Check sheet for the modelled part. Datum: model origin and axes. Units: mm. Face numbers are marked on the shaded views. Coordinates: 2 decimals unless noted, no trailing zeros. Loops run counter-clockwise (first coordinate to the right, second up) from the corner with the lowest first, then second, coordinate; pieces in that order, holes last. Notation, with made-up numbers: (-28.5, 41) - (5.5, 41) arc R18 ccw to (5.5, 58) - close; hole circle Ø8 at (19.25, 66.5). An arc over 180 degrees is marked (long way). Write each question's results on one line, items separated by ' | '. Start each with the question number.
1. Draft check along X on the marked faces 1, 2, 3 and 4. Enter one of: released by +X, released by -X, zero draft, split by the parting line, or undercut.
2. Cross-section at D-D (x = -6). Record the cut outline in (y, z), and give its area (3 significant figures).
3. Gauge pin test, flat ends, axial feed: P1, Ø1.5, axis at x = 10, z = -16.5, coming from the -Y side; P2, Ø3, axis at x = 3, z = 10.5, coming from the -Y side; P3, Ø4, axis at x = -10, z = 13, coming from the -Y side. Record the tip position at first contact, or that the pin passes through.
4. Thickness scan on line 1 (Z direction, x = 14, y = 6); line 2 (Y direction, x = 0, z = 0.5); line 3 (Y direction, x = 0, z = 17). Record the ranges inside material, lowest first. Write a range as [from, to].
5. Cross-section at C-C (z = 15). Record the cut outline in (x, y), and give its area (3 significant figures).
6. Cross-section at A-A (x = 0). Record the cut outline in (y, z).
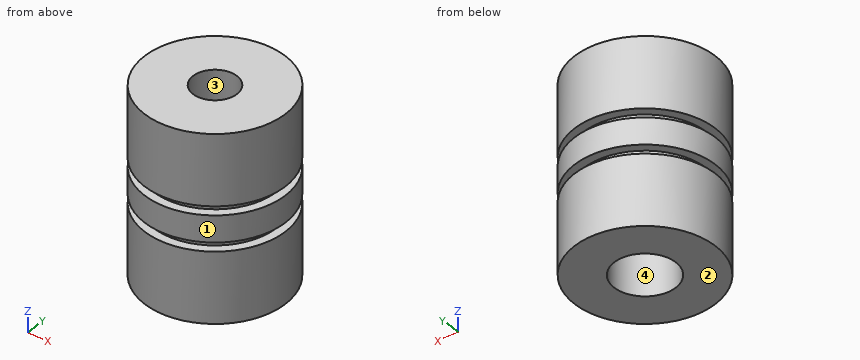
```python
from build123d import *

# Parameters (mm, degrees)
SKETCH_1_R          = 16
SKETCH_1_R_2        = 5
EXTRUDE_1_DEPTH     = 21
SKETCH_2_R          = 7
CUT_EXTRUDE_1_DEPTH = 30
CUT_EXTRUDE_START   = 5
SKETCH_3_R          = 16
SKETCH_3_R_2        = 14
CUT_EXTRUDE_3_DEPTH = 2
CUT_EXTRUDE_START_2 = -3
SKETCH_3_2_R        = 16
SKETCH_3_2_R_2      = 14
CUT_EXTRUDE_4_DEPTH = 2


with BuildPart() as part:
    # Sketch 1 → Extrude 1 (new, symmetric)
    with BuildSketch(Plane.XY):
        with Locations(Location((0, 0, 0), (0, 0, 180))):
            Circle(SKETCH_1_R)
        with Locations(Location((0, 0, 0), (0, 0, 180))):
            Circle(SKETCH_1_R_2, mode=Mode.SUBTRACT)
    extrude(amount=EXTRUDE_1_DEPTH, both=True)

    # Sketch 2 → Cut-Extrude 1 (cut)
    with BuildSketch(Plane(origin=(0, 0, -21), x_dir=(-1, 0, 0), z_dir=(0, 0, -1))):
        Circle(SKETCH_2_R)
    extrude(amount=-CUT_EXTRUDE_1_DEPTH, mode=Mode.SUBTRACT)

    # Sketch 3 → Cut-Extrude 3 (cut)
    with BuildSketch(Plane.XY.offset(CUT_EXTRUDE_START)):
        with Locations(Location((0, 0, 0), (0, 0, 180))):
            Circle(SKETCH_3_R)
        Circle(SKETCH_3_R_2, mode=Mode.SUBTRACT)
    extrude(amount=-CUT_EXTRUDE_3_DEPTH, mode=Mode.SUBTRACT)

    # Sketch 3_2 → Cut-Extrude 4 (cut)
    with BuildSketch(Plane.XY.offset(CUT_EXTRUDE_START_2)):
        with Locations(Location((0, 0, 0), (0, 0, 180))):
            Circle(SKETCH_3_2_R)
        Circle(SKETCH_3_2_R_2, mode=Mode.SUBTRACT)
    extrude(amount=-CUT_EXTRUDE_4_DEPTH, mode=Mode.SUBTRACT)


solid = part.part
```
Established:
1) face 1: split by the parting line | face 2: zero draft | face 3: undercut | face 4: undercut
2) outline: (-14.83, -21) - (-3.61, -21) - (-3.61, 9) - (3.61, 9) - (3.61, -21) - (14.83, -21) - (14.83, -5) - (12.65, -5) - (12.65, -3) - (14.83, -3) - (14.83, 3) - (12.65, 3) - (12.65, 5) - (14.83, 5) - (14.83, 21) - (-14.83, 21) - (-14.83, 5) - (-12.65, 5) - (-12.65, 3) - (-14.83, 3) - (-14.83, -3) - (-12.65, -3) - (-12.65, -5) - (-14.83, -5) - close | area: 1,010 mm^2
3) P1: y = -13.06 | P2: y = -15.93 | P3: y = -13.86
4) line 1: [-21, -5], [-3, 3], [5, 21] | line 2: [-16, -7], [7, 16] | line 3: [-16, -5], [5, 16]
5) outline: circle Ø32 at (0, 0); hole circle Ø10 at (0, 0) | area: 726 mm^2
6) outline: (-16, -21) - (-7, -21) - (-7, 9) - (-5, 9) - (-5, 21) - (-16, 21) - (-16, 5) - (-14, 5) - (-14, 3) - (-16, 3) - (-16, -3) - (-14, -3) - (-14, -5) - (-16, -5) - close; (5, 9) - (7, 9) - (7, -21) - (16, -21) - (16, -5) - (14, -5) - (14, -3) - (16, -3) - (16, 3) - (14, 3) - (14, 5) - (16, 5) - (16, 21) - (5, 21) - close
